Read the model definition and answer for the solid it produces. Units are mm, in the model's axes. A direction names the side the tool comes from. Coordinates: 2 decimals unless noted, no trailing zeros. Write each loop counter-clockwise with the first axis right and the second up, starting at its lowest first coordinate (ties: lowest second). Pieces come first, ordered by that corner, then holes. Notation, with made-up numbers: (-38.5, 75.5) -> (2.5, 75.5) arc R23 cw to (2.5, 91.5) -> close; hole circle Ø1 at (-27.75, 21.25). An arc over 180 degrees is marked (long way). One line per item, written item: value. Start each with the question number.
1. Given P1, Ø2, axis at y = 8.5, z = 108, coming from the +X side; P2, Ø1.5, axis at y = 2.5, z = 19, coming from the +X side; P3, Ø5, axis at x = -11, y = 13.5, coming from the -Z side; P4, Ø1, axis at x = 2, z = 36, coming from the +Y side, each flat-ended and moving along its own axis, determine where each tip first touches the part or whether it passes through.
2. For a pull along Z with two mould halves and no side action, classify faces 1 (the flat face through (0, 2, 83.188)), 2 (the flat face through (-22.665, 8, 104)) as pulls with the +Z half, pulls with the -Z half, needs draft (parallel to the pull), parting line crosses it, or undercut.
3. Find section D-D, the plane x = 0. State how many separate pieces and enclosed holes the cut face has, and give its area (3 significant figures).
4. For faces 3 (the cylindrical face through (13.252, 6.406, 169.106)), 4 (the flat face through (-5.225, 2.537, 124.324)), 5 (the flat face through (10.179, 4.506, 84.18)), 6 (the flat face through (-15.577, 11.204, 17.531)), determine the directions among +Z, -Z, +X, -X, +Y, -Y from which every point of the face is accessible in a straight line to the end or side of a thin tool.
5. Find section C-C, the plane z = 38. Write down the section's boundary in (x, y), and give its area (3 significant figures).
6. Find section A-A, the plane x = -16. Write down the section's boundary in (y, z), and give its area (3 significant figures).
7. Consider line 1 along X through (y, z) = (6.75, 9); line 2 along Z through (x, y) = (12, 11.25); line 3 along X through (y, z) = (11, 169). Determine where each line is inside the solid, lowest interval first.
```python
from build123d import *

# Parameters (mm, degrees)
SKETCH242_AS_DRAWN_R                    = 1.85
EXTRUDE136028_DEPTH                     = 20
EXTRUDE136028_ONTO_SKETCH242_ROLL_ANGLE = 90
EXTRUDE136035_DEPTH                     = 50
SKETCH245_AS_DRAWN_R                    = 2.75
EXTRUDE136031_DEPTH                     = 9
EXTRUDE136031_ONTO_SKETCH245_ROLL_ANGLE = 90
SKETCH244_AS_DRAWN_R                    = 1.85
EXTRUDE136030_DEPTH                     = 20
EXTRUDE136030_ONTO_SKETCH244_ROLL_ANGLE = 90
EXTRUDE136029_DEPTH                     = 38
EXTRUDE136036_DEPTH                     = 50
SKETCH248_AS_DRAWN_R                    = 2.75
EXTRUDE136034_DEPTH                     = 9
EXTRUDE136034_ONTO_SKETCH248_ROLL_ANGLE = 90
SKETCH247_AS_DRAWN_R                    = 1.85
EXTRUDE136033_DEPTH                     = 20
EXTRUDE136033_ONTO_SKETCH247_ROLL_ANGLE = 90
EXTRUDE136032_DEPTH                     = 24
EXTRUDE136037_DEPTH                     = 14
SKETCH252_W                             = 9.75
SKETCH252_H                             = 16.75
EXTRUDE136038_DEPTH                     = 9
EXTRUDE136039_DEPTH                     = 7
EXTRUDE136027_DEPTH                     = 135


with BuildPart() as extrude136028:
    # Sketch242 as drawn → Extrude136028 (new)
    with BuildSketch(Plane.XY):
        with Locations((0, -9)):
            Circle(SKETCH242_AS_DRAWN_R)
        Polygon((3.5, 19.187822), (7, 25.25), (3.5, 31.312178), (-3.5, 31.312178), (-7, 25.25), (-3.5, 19.187822), align=None)
        Polygon((3.5, 35.187822), (7, 41.25), (3.5, 47.312178), (-3.5, 47.312178), (-7, 41.25), (-3.5, 35.187822), align=None)
        Polygon((3.5, 51.187822), (7, 57.25), (3.5, 63.312178), (-3.5, 63.312178), (-7, 57.25), (-3.5, 51.187822), align=None)
        Polygon((3.5, 67.187822), (7, 73.25), (3.5, 79.312178), (-3.5, 79.312178), (-7, 73.25), (-3.5, 67.187822), align=None)
        Polygon((3.5, 83.187822), (7, 89.25), (3.5, 95.312178), (-3.5, 95.312178), (-7, 89.25), (-3.5, 83.187822), align=None)
        Polygon((3.5, 99.187822), (7, 105.25), (3.5, 111.312178), (-3.5, 111.312178), (-7, 105.25), (-3.5, 99.187822), align=None)
        Polygon((3.5, 115.187822), (7, 121.25), (3.5, 127.312178), (-3.5, 127.312178), (-7, 121.25), (-3.5, 115.187822), align=None)
        Polygon((3.5, 131.187822), (7, 137.25), (3.5, 143.312178), (-3.5, 143.312178), (-7, 137.25), (-3.5, 131.187822), align=None)
        with BuildLine():
            Line((5, -8.999981), (5, -15.999981))
            Line((5, -15.999981), (-5, -15.999981))
            Line((-5, -15.999981), (-5, -8.999981))
            ThreePointArc((-5, -8.999981), (0, -14), (5, -8.999981))
        make_face()
    extrude(amount=-EXTRUDE136028_DEPTH)


with BuildPart() as extrude136028_1:
    # Extrude136028 onto Sketch242 roll: moved
    add(extrude136028.part.rotate(Axis((0, 0, 0), (1, 0, 0)), EXTRUDE136028_ONTO_SKETCH242_ROLL_ANGLE))


with BuildPart() as extrude136028_2:
    # Extrude136028 onto Sketch242 placement: moved
    add(extrude136028_1.part)


with BuildPart() as extrude136035:
    # Sketch249 → Extrude136035 (new body)
    with BuildSketch(Plane.YZ):
        Polygon((0, -9.814955), (17, 0), (17, -9.814955), align=None)
        Polygon((17, 29), (0, 19.185045), (0, 29), align=None)
    extrude(amount=EXTRUDE136035_DEPTH)


with BuildPart() as extrude136035_1:
    # Extrude136035 placement: moved
    add(extrude136035.part.moved(Location((-25, 0, 0))))


with BuildPart() as extrude136031:
    # Sketch245 as drawn → Extrude136031 (new)
    with BuildSketch(Plane.XY):
        with Locations((-16, 0)):
            Circle(SKETCH245_AS_DRAWN_R)
        with Locations((16, 0)):
            Circle(SKETCH245_AS_DRAWN_R)
    extrude(amount=-EXTRUDE136031_DEPTH)


with BuildPart() as extrude136031_1:
    # Extrude136031 onto Sketch245 roll: moved
    add(extrude136031.part.rotate(Axis((0, 0, 0), (1, 0, 0)), EXTRUDE136031_ONTO_SKETCH245_ROLL_ANGLE))


with BuildPart() as extrude136031_2:
    # Extrude136031 onto Sketch245 placement: moved
    add(extrude136031_1.part)


with BuildPart() as fusion034004041043:
    # Sketch244 as drawn → Extrude136030 (new)
    with BuildSketch(Plane.XY):
        with Locations((-16, 0)):
            Circle(SKETCH244_AS_DRAWN_R)
        with Locations((16, 0)):
            Circle(SKETCH244_AS_DRAWN_R)
    extrude(amount=-EXTRUDE136030_DEPTH)


with BuildPart() as fusion034004041043_1:
    # Extrude136030 onto Sketch244 roll: moved
    add(fusion034004041043.part.rotate(Axis((0, 0, 0), (1, 0, 0)), EXTRUDE136030_ONTO_SKETCH244_ROLL_ANGLE))


with BuildPart() as fusion034004041043_2:
    # Extrude136030 onto Sketch244 placement: moved
    add(fusion034004041043_1.part)

    # Fusion034004041041: union Extrude136031
    add(extrude136031_2.part)


with BuildPart() as fusion034004041043_3:
    # Fusion034004041041 placement: moved
    add(fusion034004041043_2.part.moved(Location((0, 0, 13))))

    # Fusion034004041043: union Extrude136035
    add(extrude136035_1.part)


with BuildPart() as cut009010006006006005003:
    # Sketch243 → Extrude136029 (new body)
    with BuildSketch(Plane.XY):
        with BuildLine():
            Line((-11, 0), (11, 0))
            Line((20.5, 11.321659), (11, 0))
            Line((20.5, 11.321659), (20.5, 16.890918))
            Line((20.5, 16.890918), (12.499524, 16.890918))
            ThreePointArc((-12.499524, 16.890918), (0, 4.5), (12.499524, 16.890918))
            Line((-20.5, 16.890918), (-12.499524, 16.890918))
            Line((-20.5, 11.321659), (-20.5, 16.890918))
            Line((-20.5, 11.321659), (-11, 0))
        make_face()
    extrude(amount=EXTRUDE136029_DEPTH)


with BuildPart() as cut009010006006006005003_1:
    # Extrude136029 placement: moved
    add(cut009010006006006005003.part.moved(Location((0, 0, -9))))

    # Cut009010006006006005003: cut Fusion034004041043
    add(fusion034004041043_3.part, mode=Mode.SUBTRACT)


with BuildPart() as cut009010006006006005003_2:
    # Cut009010006006006005003 placement: moved
    add(cut009010006006006005003_1.part.moved(Location((0, 0, 156))))


with BuildPart() as extrude136036:
    # Sketch250 → Extrude136036 (new body)
    with BuildSketch(Plane.YZ):
        Polygon((0, 24), (17, 24), (17, 14.185045), align=None)
    extrude(amount=EXTRUDE136036_DEPTH)


with BuildPart() as extrude136036_1:
    # Extrude136036 placement: moved
    add(extrude136036.part.moved(Location((-25, 0, 0))))


with BuildPart() as extrude136034:
    # Sketch248 as drawn → Extrude136034 (new)
    with BuildSketch(Plane.XY):
        with Locations((-16, 0)):
            Circle(SKETCH248_AS_DRAWN_R)
        with Locations((16, 0)):
            Circle(SKETCH248_AS_DRAWN_R)
    extrude(amount=-EXTRUDE136034_DEPTH)


with BuildPart() as extrude136034_1:
    # Extrude136034 onto Sketch248 roll: moved
    add(extrude136034.part.rotate(Axis((0, 0, 0), (1, 0, 0)), EXTRUDE136034_ONTO_SKETCH248_ROLL_ANGLE))


with BuildPart() as extrude136034_2:
    # Extrude136034 onto Sketch248 placement: moved
    add(extrude136034_1.part)


with BuildPart() as fusion034004041042:
    # Sketch247 as drawn → Extrude136033 (new)
    with BuildSketch(Plane.XY):
        with Locations((-16, 0)):
            Circle(SKETCH247_AS_DRAWN_R)
        with Locations((16, 0)):
            Circle(SKETCH247_AS_DRAWN_R)
    extrude(amount=-EXTRUDE136033_DEPTH)


with BuildPart() as fusion034004041042_1:
    # Extrude136033 onto Sketch247 roll: moved
    add(fusion034004041042.part.rotate(Axis((0, 0, 0), (1, 0, 0)), EXTRUDE136033_ONTO_SKETCH247_ROLL_ANGLE))


with BuildPart() as fusion034004041042_2:
    # Extrude136033 onto Sketch247 placement: moved
    add(fusion034004041042_1.part)

    # Fusion034004041042: union Extrude136034
    add(extrude136034_2.part)


with BuildPart() as fusion034004041042_3:
    # Fusion034004041042 placement: moved
    add(fusion034004041042_2.part.moved(Location((0, 0, 9))))


with BuildPart() as cut009010006006006005004:
    # Sketch246 → Extrude136032 (new body)
    with BuildSketch(Plane.XY):
        with BuildLine():
            Line((-11, 0), (11, 0))
            Line((20.5, 11.321659), (11, 0))
            Line((20.5, 11.321659), (20.5, 16.890918))
            Line((20.5, 16.890918), (12.499524, 16.890918))
            ThreePointArc((-12.499524, 16.890918), (0, 4.5), (12.499524, 16.890918))
            Line((-20.5, 16.890918), (-12.499524, 16.890918))
            Line((-20.5, 11.321659), (-20.5, 16.890918))
            Line((-20.5, 11.321659), (-11, 0))
        make_face()
    extrude(amount=EXTRUDE136032_DEPTH)

    # Cut009010006006006005002: cut Fusion034004041042
    add(fusion034004041042_3.part, mode=Mode.SUBTRACT)

    # Cut009010006006006005004: cut Extrude136036
    add(extrude136036_1.part, mode=Mode.SUBTRACT)


with BuildPart() as extrude136037:
    # Sketch251 → Extrude136037 (new body)
    with BuildSketch(Plane.XY):
        with BuildLine():
            Line((-4.875, 0), (4.875, 0))
            Line((4.875, 5.489814), (4.875, 0))
            ThreePointArc((-4.875, 5.489814), (0, 4.5), (4.875, 5.489814))
            Line((-4.875, 5.489814), (-4.875, 0))
        make_face()
    extrude(amount=-EXTRUDE136037_DEPTH)


with BuildPart() as extrude136038:
    # Sketch252 → Extrude136038 (new body)
    with BuildSketch(Plane.XY):
        with Locations((0, 8.375)):
            Rectangle(SKETCH252_W, SKETCH252_H)
    extrude(amount=-EXTRUDE136038_DEPTH)


with BuildPart() as extrude136038_1:
    # Extrude136038 placement: moved
    add(extrude136038.part.moved(Location((0, 0, -5))))


with BuildPart() as extrude136039:
    # Sketch253 → Extrude136039 (new body)
    with BuildSketch(Plane.XY):
        Polygon((0, 5), (0, 0), (-20.5, 0), (-22.665064, 3.75), (-22.665064, 11.75), (-20.5, 15.5), (-18, 15.5), (-18, 13), (-18.665064, 11.848076), (-18.665064, 6.151924), (-18, 5), align=None)
    extrude(amount=EXTRUDE136039_DEPTH)


with BuildPart() as extrude136039_1:
    # Extrude136039 placement: moved
    add(extrude136039.part.moved(Location((0, 0, 101))))


with BuildPart() as cut009010006006006005005:
    # Sketch241 → Extrude136027 (new body)
    with BuildSketch(Plane.XY):
        with BuildLine():
            Line((-11, 0), (11, 0))
            Line((11, 0), (12.678199, 2))
            Line((12.678199, 2), (7.609518, 7.083083))
            ThreePointArc((-7.609518, 7.083083), (0, 4.5), (7.609518, 7.083083))
            Line((-12.678199, 2), (-7.609518, 7.083083))
            Line((-11, 0), (-12.678199, 2))
        make_face()
    extrude(amount=EXTRUDE136027_DEPTH)


with BuildPart() as cut009010006006006005005_1:
    # Extrude136027 placement: moved
    add(cut009010006006006005005.part.moved(Location((0, 0, 17))))

    # Fusion034004041027: union Cut009010006006006005003, Cut009010006006006005004, Extrude136037, Extrude136038, Extrude136039
    add(cut009010006006006005003_2.part)
    add(cut009010006006006005004.part)
    add(extrude136037.part)
    add(extrude136038_1.part)
    add(extrude136039_1.part)

    # Cut009010006006006005005: cut Extrude136028
    add(extrude136028_2.part, mode=Mode.SUBTRACT)


solid = cut009010006006006005005_1.part
```
Answer block:
1. P1: stops at x = -18.67
1. P2: stops at x = 13.73
1. P3: stops at z = 0
1. P4: passes through
2. face 1: undercut
2. face 2: needs draft
3. separate pieces: 10
3. enclosed holes: 0
3. area: 469 mm2
4. face 3: -Y
4. face 4: +Y, -Y
4. face 5: +X, +Y
4. face 6: -X, +Y
5. outline: (-12.68, 2) -> (-11, 0) -> (-5.12, 0) -> (-5.12, 5.6) arc R12.5 cw to (-7.61, 7.08) -> close; (5.12, 0) -> (11, 0) -> (12.68, 2) -> (7.61, 7.08) arc R12.5 cw to (5.12, 5.6) -> close
5. area: 73.9 mm2
6. outline: (0, 101) -> (5, 101) -> (5, 108) -> (0, 108) -> close; (5.96, 0) -> (16.89, 0) -> (16.89, 7.15) -> (9, 7.15) -> (9, 6.25) -> (5.96, 6.25) -> close; (5.96, 11.75) -> (9, 11.75) -> (9, 10.85) -> (16.89, 10.85) -> (16.89, 14.25) -> (5.96, 20.56) -> close; (5.96, 149.63) -> (16.89, 155.94) -> (16.89, 167.15) -> (9, 167.15) -> (9, 166.25) -> (5.96, 166.25) -> close; (5.96, 171.75) -> (9, 171.75) -> (9, 170.85) -> (16.89, 170.85) -> (16.89, 184.94) -> (5.96, 178.63) -> close
6. area: 450 mm2
7. line 1: x = -13.25 to -7.15, 7.15 to 13.25
7. line 2: z = 0 to 17.5, 152.68 to 181.68
7. line 3: x = -20.23 to -17.85, -14.15 to -10.97, 10.97 to 14.15, 17.85 to 20.23
